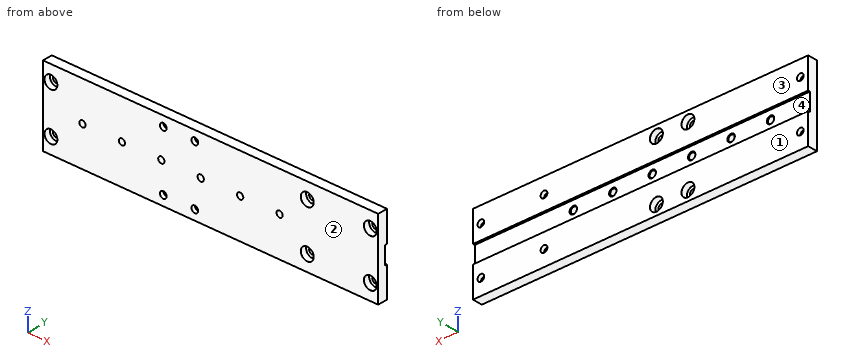
from build123d import *

# Parameters (mm, degrees)
ESBO_O1_W                                         = 170
ESBO_O1_H                                         = 40
RESSALTO_EXTRUS_O1_DEPTH                          = 5
ESBO_O2_W                                         = 170
ESBO_O2_H                                         = 9
CORTE_EXTRUS_O1_DEPTH                             = 1
REBAIXO_PARA_SHCS_M31_AT_2_COUNT                  = 2
REBAIXO_PARA_SHCS_M31_AT_2_PITCH                  = 24
REBAIXO_PARA_SHCS_M31_AT_3_COUNT                  = 2
REBAIXO_PARA_SHCS_M31_AT_3_PITCH                  = 130
REBAIXO_PARA_SHCS_M31_AT_4_COUNT                  = 2
REBAIXO_PARA_SHCS_M31_AT_4_PITCH                  = 132.196822957
REBAIXO_PARA_SHCS_M31_AT_5_COUNT                  = 2
REBAIXO_PARA_SHCS_M31_AT_5_PITCH                  = 162
REBAIXO_PARA_SHCS_M31_AT_6_COUNT                  = 2
REBAIXO_PARA_SHCS_M31_AT_6_PITCH                  = 163.768128767
REBAIXO_PARA_SHCS_M32_AT_2_COUNT                  = 2
REBAIXO_PARA_SHCS_M32_AT_2_PITCH                  = 16
REBAIXO_PARA_SHCS_M32_AT_3_COUNT                  = 2
REBAIXO_PARA_SHCS_M32_AT_3_PITCH                  = 30
REBAIXO_PARA_SHCS_M32_AT_4_COUNT                  = 2
REBAIXO_PARA_SHCS_M32_AT_4_PITCH                  = 34
FURO_ROSCADO_PARA_CONDU_TE_DE_M3X0_51_D           = 3.15
FURO_ROSCADO_PARA_CONDU_TE_DE_M3X0_51_CSINK_D     = 3.766
FURO_ROSCADO_PARA_CONDU_TE_DE_M3X0_51_CSINK_ANGLE = 90


with BuildPart() as part:
    # Esboço1 → Ressalto-extrusão1 (new body)
    with BuildSketch(Plane(origin=(0, 0, 0), x_dir=(1, 0, 0), z_dir=(0, 1, 0))):
        Rectangle(ESBO_O1_W, ESBO_O1_H)
    extrude(amount=RESSALTO_EXTRUS_O1_DEPTH)

    # Esboço2 → Corte-extrusão1 (cut)
    with BuildSketch(Plane(origin=(0, 5, 0), x_dir=(1, 0, 0), z_dir=(0, 1, 0))):
        Rectangle(ESBO_O2_W, ESBO_O2_H)
    extrude(amount=-CORTE_EXTRUS_O1_DEPTH, mode=Mode.SUBTRACT)

    # Esboço4 → Rebaixo para SHCS M31 (revolve, cut)
    with BuildSketch(Plane(origin=(-81, 0, -12), x_dir=(0, 0, -1), z_dir=(1, 0, 0))):
        Polygon((0, 0), (0, 5), (1.7, 5), (1.7, 3), (3.25, 3), (3.25, 0.025), (3.275, 0), align=None)
    rebaixo_para_shcs_m31 = revolve(axis=Axis((-81, -6.35, -12), (0, 1, 0)), mode=Mode.SUBTRACT)

    # Rebaixo para SHCS M31 at 2: Rebaixo para SHCS M31 ×2
    with Locations(*[(0, 0, i * REBAIXO_PARA_SHCS_M31_AT_2_PITCH) for i in range(1, REBAIXO_PARA_SHCS_M31_AT_2_COUNT)]):
        add(rebaixo_para_shcs_m31, mode=Mode.SUBTRACT)

    # Rebaixo para SHCS M31 at 3: Rebaixo para SHCS M31 ×2
    with Locations(*[(i * REBAIXO_PARA_SHCS_M31_AT_3_PITCH, 0, 0) for i in range(1, REBAIXO_PARA_SHCS_M31_AT_3_COUNT)]):
        add(rebaixo_para_shcs_m31, mode=Mode.SUBTRACT)

    # Rebaixo para SHCS M31 at 4: Rebaixo para SHCS M31 ×2
    with Locations(*[Vector(0.98338218, 0, 0.181547479) * (i * REBAIXO_PARA_SHCS_M31_AT_4_PITCH) for i in range(1, REBAIXO_PARA_SHCS_M31_AT_4_COUNT)]):
        add(rebaixo_para_shcs_m31, mode=Mode.SUBTRACT)

    # Rebaixo para SHCS M31 at 5: Rebaixo para SHCS M31 ×2
    with Locations(*[(i * REBAIXO_PARA_SHCS_M31_AT_5_PITCH, 0, 0) for i in range(1, REBAIXO_PARA_SHCS_M31_AT_5_COUNT)]):
        add(rebaixo_para_shcs_m31, mode=Mode.SUBTRACT)

    # Rebaixo para SHCS M31 at 6: Rebaixo para SHCS M31 ×2
    with Locations(*[Vector(0.989203462, 0, 0.146548661) * (i * REBAIXO_PARA_SHCS_M31_AT_6_PITCH) for i in range(1, REBAIXO_PARA_SHCS_M31_AT_6_COUNT)]):
        add(rebaixo_para_shcs_m31, mode=Mode.SUBTRACT)

    # Esboço6 → Rebaixo para SHCS M32 (revolve, cut)
    with BuildSketch(Plane(origin=(-24, 5, -15), x_dir=(0, 0, 1), z_dir=(1, 0, 0))):
        Polygon((0, 0), (0, 5), (1.7, 5), (1.7, 3), (3.25, 3), (3.25, 0.025), (3.275, 0), align=None)
    rebaixo_para_shcs_m32 = revolve(axis=Axis((-24, 11.35, -15), (0, -1, 0)), mode=Mode.SUBTRACT)

    # Rebaixo para SHCS M32 at 2: Rebaixo para SHCS M32 ×2
    with Locations(*[(i * REBAIXO_PARA_SHCS_M32_AT_2_PITCH, 0, 0) for i in range(1, REBAIXO_PARA_SHCS_M32_AT_2_COUNT)]):
        add(rebaixo_para_shcs_m32, mode=Mode.SUBTRACT)

    # Rebaixo para SHCS M32 at 3: Rebaixo para SHCS M32 ×2
    with Locations(*[(0, 0, i * REBAIXO_PARA_SHCS_M32_AT_3_PITCH) for i in range(1, REBAIXO_PARA_SHCS_M32_AT_3_COUNT)]):
        add(rebaixo_para_shcs_m32, mode=Mode.SUBTRACT)

    # Rebaixo para SHCS M32 at 4: Rebaixo para SHCS M32 ×2
    with Locations(*[Vector(0.470588235, 0, 0.882352941) * (i * REBAIXO_PARA_SHCS_M32_AT_4_PITCH) for i in range(1, REBAIXO_PARA_SHCS_M32_AT_4_COUNT)]):
        add(rebaixo_para_shcs_m32, mode=Mode.SUBTRACT)

    # Furo roscado para conduíte de M3x0.51 (through all)
    with Locations(Plane(origin=(0, 4, 0), x_dir=(1, 0, 0), z_dir=(0, 1, 0))):
        with Locations((-65, 0), (-45, 0), (-25, 0), (35, 0), (-5, 0), (15, 0)):
            CounterSinkHole(FURO_ROSCADO_PARA_CONDU_TE_DE_M3X0_51_D / 2, FURO_ROSCADO_PARA_CONDU_TE_DE_M3X0_51_CSINK_D / 2, counter_sink_angle=FURO_ROSCADO_PARA_CONDU_TE_DE_M3X0_51_CSINK_ANGLE)


solid = part.part
Geometry: final body of the model. Coordinates: model frame, mm. Face numbers are marked on the shaded views. A direction names the side the tool comes from. Give positions to 0.01 mm unless a question says otherwise; leave off trailing zeros. Write each loop counter-clockwise with the first axis right and the second up, starting at its lowest first coordinate (ties: lowest second). Pieces come first, ordered by that corner, then holes. Notation, with made-up numbers: (53.5, 51) -> (75.5, 51) arc R8 ccw to (75.5, 56) -> close; hole circle Ø11 at (-4.5, -26). An arc over 180 degrees is marked (long way). Answer in a Markdown table with one row per item.
(1) Section query B-B on x = -37.5. Return loops of the section in (y, z).
Answers below:
| item | result |
|---|---|
| outline | (0, -20) -> (5, -20) -> (5, -4.5) -> (4, -4.5) -> (4, 4.5) -> (5, 4.5) -> (5, 20) -> (0, 20) -> close |
(2) Section query A-A on x = 49. Return loops of the section in (y, z) (3 decimals), then the cut area to 3 significant figures.
Answers below:
| item | result |
|---|---|
| outline | (0, -20) -> (5, -20) -> (5, -13.7) -> (3, -13.7) -> (3, -15.25) -> (0.025, -15.25) -> (0, -15.275) -> close; (0, -8.725) -> (0.025, -8.75) -> (3, -8.75) -> (3, -10.3) -> (5, -10.3) -> (5, -4.5) -> (4, -4.5) -> (4, 4.5) -> (5, 4.5) -> (5, 10.3) -> (3, 10.3) -> (3, 8.75) -> (0.025, 8.75) -> (0, 8.725) -> close; (0, 15.275) -> (0.025, 15.25) -> (3, 15.25) -> (3, 13.7) -> (5, 13.7) -> (5, 20) -> (0, 20) -> close |
| area | 138 mm^2 |
(3) Ray query, line 1 along X through (y, z) = (3.75, 15); line 2 along Z through (x, y) = (49, 3.7); line 3 along X through (y, z) = (2.9, 17.5). Return the intervals inside material, ascending. Write a range as [from, to].
Answers below:
| item | result |
|---|---|
| line 1 | [-85, -27.25], [-20.75, -11.25], [-4.75, 85] |
| line 2 | [-20, -13.7], [-10.3, 10.3], [13.7, 20] |
| line 3 | [-85, -26.08], [-21.92, -10.08], [-5.92, 85] |
(4) Draft query along Y for the marked faces 1 and 2. Return one class per face: +Y half, -Y half, draft (parallel to the pull), parting line (faces both ways), or undercut.
Answers below:
| item | result |
|---|---|
| face 1 | +Y half |
| face 2 | -Y half |
(5) Pin query (flat end, axial travel): pin 1 (2.5 mm diameter, centred on x = -8, z = 15, fed in from -Y); pin 2 (5 mm diameter, centred on x = 3, z = -3, fed in from -Y); pin 3 (4 mm diameter, centred on x = -81, z = -12, fed in from -Y); pin 4 (2 mm diameter, centred on x = -25, z = 16, fed in from +Y). Return the tip coordinate at first contact, or that it passes through.
Answers below:
| item | result |
|---|---|
| pin 1 | through |
| pin 2 | y = 0 |
| pin 3 | y = 3 |
| pin 4 | y = 2 |
(6) Set-up query: the marked faces 3 and 4. Return all of +Z, -Z, +X, -X, +Y, -Y with unobstructed straight access to the full face (end or side cutting, diameter ignored); none if empty.
Answers below:
| item | result |
|---|---|
| face 3 | +Z, -Z, +X, -X, +Y |
| face 4 | +X, -X, +Y |
